from build123d import *

# Parameters (mm, degrees)
F0_W     = 29
F0_H     = 152
F1_DEPTH = 26
F2_R     = 3
F2_R_2   = 2.75
F3_DEPTH = 26.001
F4_W     = 23
F4_H     = 67
F4_R     = 3
F5_DEPTH = 19.2
F6_W     = 10
F6_H     = 8
F6_R     = 3
F7_DEPTH = 2
F8_W     = 29
F8_H     = 40
F8_R     = 3
F9_DEPTH = 4.4


with BuildPart() as f1:
    # F0 (on Top) → F1 (new body)
    with BuildSketch(Plane.XY):
        Rectangle(F0_W, F0_H)
    extrude(amount=F1_DEPTH)

    # F2 (on face) → F3 (cut, through all)
    with BuildSketch(Plane.XY.offset(26)):
        with Locations((0, -60)):
            Circle(F2_R)
        with Locations((0, 60)):
            Circle(F2_R_2)
    extrude(amount=-F3_DEPTH, mode=Mode.SUBTRACT)

    # F4 (on face) → F5 (cut)
    with BuildSketch(Plane.XY.offset(26)):
        with Locations((0, -38.5)):
            Rectangle(F4_W, F4_H)
        with Locations((0, -60)):
            Circle(F4_R, mode=Mode.SUBTRACT)
    extrude(amount=-F5_DEPTH, mode=Mode.SUBTRACT)

    # F6 (on face) → F7 (cut)
    with BuildSketch(Plane.XY.offset(6.8)):
        with Locations((0, -28)):
            Rectangle(F6_W, F6_H)
        with Locations((0, -49)):
            Circle(F6_R)
    extrude(amount=-F7_DEPTH, mode=Mode.SUBTRACT)

    # F8 (on face) → F9 (cut)
    with BuildSketch(Plane(origin=(0, 0, 0), x_dir=(1, 0, 0), z_dir=(0, 0, -1))):
        with Locations((0, 56)):
            Rectangle(F8_W, F8_H)
        with Locations((0, 60)):
            Circle(F8_R, mode=Mode.SUBTRACT)
        with BuildLine():
            ThreePointArc((-14.5, 6), (-2.691813, 23.602086), (14.5, 36))
            Line((14.5, 36), (-14.5, 36))
            Line((-14.5, 36), (-14.5, 6))
        make_face()
    extrude(amount=-F9_DEPTH, mode=Mode.SUBTRACT)


solid = f1.part
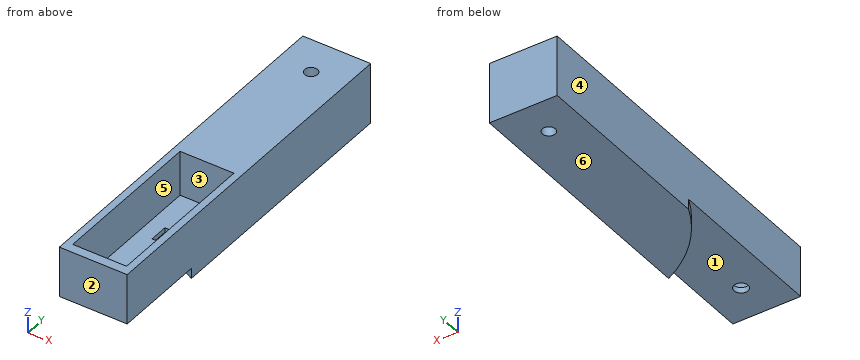
Read the model definition and answer for the solid it produces. Units are mm, in the model's axes. Face numbers are marked on the shaded views. A direction names the side the tool comes from. Coordinates: 2 decimals unless noted, no trailing zeros. Loops run counter-clockwise (first coordinate to the right, second up) from the corner with the lowest first, then second, coordinate; pieces in that order, holes last. Notation, with made-up numbers: (31.25, 66) -> (36.25, 66) arc R25 cw to (36.25, 103) -> close; hole circle Ø2 at (-15, 6.5). An arc over 180 degrees is marked (long way). Answer in a Markdown table with one row per item.
Item 1: A cutting plane is placed at D-D on x = 0. Determine the outline of the cut face in (y, z).
Returned:
| item | result |
|---|---|
| outline | (-76, 4.4) -> (-63, 4.4) -> (-63, 6.8) -> (-72, 6.8) -> (-72, 26) -> (-76, 26) -> close; (-57, 4.4) -> (-26.22, 4.4) -> (-26.22, 0) -> (57.25, 0) -> (57.25, 26) -> (-5, 26) -> (-5, 6.8) -> (-24, 6.8) -> (-24, 4.8) -> (-32, 4.8) -> (-32, 6.8) -> (-46, 6.8) -> (-46, 4.8) -> (-52, 4.8) -> (-52, 6.8) -> (-57, 6.8) -> close; (62.75, 0) -> (76, 0) -> (76, 26) -> (62.75, 26) -> close |
Item 2: Straight lines are drawn through the part: line 1 along Y through (x, z) = (0, 5.95); line 2 along Y through (x, z) = (-0.25, 14.25); line 3 along Y through (x, z) = (8.75, 22.5). For each, find the intervals that lie inside material, in ascending order. Write a range as [from, to].
Returned:
| item | result |
|---|---|
| line 1 | y = [-76, -63], [-57, -52], [-46, -32], [-24, 57.25], [62.75, 76] |
| line 2 | y = [-76, -72], [-5, 57.26], [62.74, 76] |
| line 3 | y = [-76, -72], [-5, 76] |
Item 3: A cutting plane is placed at B-B on z = 16.25. Determine the outline of the cut face in (x, y).
Returned:
| item | result |
|---|---|
| outline | (-14.5, -76) -> (14.5, -76) -> (14.5, 76) -> (-14.5, 76) -> close; hole (-11.5, -72) -> (11.5, -72) -> (11.5, -5) -> (-11.5, -5) -> close; hole circle Ø5.5 at (0, 60) |
Item 4: A cutting plane is placed at A-A on y = 60. Determine the outline of the cut face in (x, z).
Returned:
| item | result |
|---|---|
| outline | (-14.5, 0) -> (-2.75, 0) -> (-2.75, 26) -> (-14.5, 26) -> close; (2.75, 0) -> (14.5, 0) -> (14.5, 26) -> (2.75, 26) -> close |
Item 5: Each of these flat-tipped pins is pushed along its axis until it touches: P1, Ø9, axis at x = 1, y = -26.5, coming from the +Z side; P2, Ø2, axis at x = -6, y = 14.5, coming from the -Z side; P3, Ø3, axis at x = 0.5, y = -48, coming from the +Z side. Where does it stop, or does it pass through?
Returned:
| item | result |
|---|---|
| P1 | stops at z = 6.8 |
| P2 | stops at z = 0 |
| P3 | stops at z = 4.8 |
Item 6: For a pull along X with two mould halves and no side action, classify the marked faces 4, 5 and 6 as released by +X, released by -X, zero draft, split by the parting line, or undercut.
Returned:
| item | result |
|---|---|
| face 4 | released by -X |
| face 5 | undercut |
| face 6 | zero draft |
Item 7: A cutting plane is placed at C-C on y = -49. Determine the outline of the cut face in (x, z).
Returned:
| item | result |
|---|---|
| outline | (-14.5, 4.4) -> (14.5, 4.4) -> (14.5, 26) -> (11.5, 26) -> (11.5, 6.8) -> (3, 6.8) -> (3, 4.8) -> (-3, 4.8) -> (-3, 6.8) -> (-11.5, 6.8) -> (-11.5, 26) -> (-14.5, 26) -> close |
Item 8: For the marked faces 1, 2 and 3, determine the directions among +Z, -Z, +X, -X, +Y, -Y from which every point of the face is accessible in a straight line to the end or side of a thin tool.
Returned:
| item | result |
|---|---|
| face 1 | -Z, -X, -Y |
| face 2 | +Z, -Z, +X, -X, -Y |
| face 3 | +Z |
